from build123d import *

# Parameters (mm, degrees)
PAD_DEPTH    = 6
SKETCH002_R  = 4.2
POCKET_DEPTH = 59.001
CHAMFER_SIZE = 5
FILLET_R     = 16


with BuildPart() as part:
    # Sketch → Pad (new body, symmetric)
    with BuildSketch(Plane.XY):
        with BuildLine():
            Line((20.75, -22.5), (20.75, 22.5))
            Line((20.75, 22.5), (-20.75, 22.5))
            ThreePointArc((-20.75, 22.5), (-33.124369, 17.374369), (-38.25, 5))
            Line((-38.25, 5), (-38.25, -5))
            ThreePointArc((-38.25, -5), (-33.124369, -17.374369), (-20.75, -22.5))
            Line((20.75, -22.5), (-20.75, -22.5))
        make_face()
    extrude(amount=PAD_DEPTH, both=True)

    # Sketch002 → Pocket (cut, through all)
    with BuildSketch(Plane.YZ.offset(20.75)):
        Circle(SKETCH002_R)
    extrude(amount=-POCKET_DEPTH, mode=Mode.SUBTRACT)

    # Chamfer
    chamfer_edges = [part.edges().sort_by_distance(p)[0] for p in [
        (20.75, 22.5, 0),
        (20.75, -22.5, 0),
    ]]
    chamfer(chamfer_edges, length=CHAMFER_SIZE)

    # Fillet
    fillet_edges = [part.edges().sort_by_distance(p)[0] for p in [
        (15.75, 22.5, 0),
        (15.75, -22.5, 0),
    ]]
    fillet(fillet_edges, radius=FILLET_R)


solid = part.part
Read the model definition and answer for the solid it produces. Units are mm, in the model's axes. Coordinates: 2 decimals unless noted, no trailing zeros. Write each loop counter-clockwise with the first axis right and the second up, starting at its lowest first coordinate (ties: lowest second). Pieces come first, ordered by that corner, then holes. Notation, with made-up numbers: (24.5, 53.5) - (80.5, 53.5) arc R8 ccw to (80.5, 58.5) - close; hole circle Ø9 at (35, -36.75). An arc over 180 degrees is marked (long way). One line per question, with ' | ' between items.
Q1. Find section A-A, the plane y = 0. Write down the section's boundary in (x, z), plus the area to 3 significant figures.
Result set:
outline: (-38.25, -6) - (20.75, -6) - (20.75, -4.2) - (-38.25, -4.2) - close; (-38.25, 4.2) - (20.75, 4.2) - (20.75, 6) - (-38.25, 6) - close | area: 212 mm^2
Q2. Find section B-B, the plane z = 0. Write down the section's boundary in (x, y), plus the area to 3 significant figures.
Result set:
outline: (-38.25, -5) arc R17.5 ccw to (-20.75, -22.5) - (9.12, -22.5) arc R16 ccw to (20.44, -17.81) - (20.75, -17.5) - (20.75, -4.2) - (-38.25, -4.2) - close; (-38.25, 4.2) - (20.75, 4.2) - (20.75, 17.5) - (20.44, 17.81) arc R16 ccw to (9.12, 22.5) - (-20.75, 22.5) arc R17.5 ccw to (-38.25, 5) - close | area: 1,990 mm^2
Q3. Consider L1, parallel to Z at x = -12.5, y = 0; L2, parallel to Y at x = 17, z = 2; L3, parallel to Y at x = -32, z = -1.75. Determine where each line is inside the solid, lowest interval first. Write a range as [from, to].
Result set:
L1: [-6, -4.2], [4.2, 6] | L2: [-20.43, -3.69], [3.69, 20.43] | L3: [-18.4, -3.82], [3.82, 18.4]
Q4. Determine the mould class of faces 1 (the cylindrical face through (15.327, -21.248, -0.084)), 2 (the flat face through (-6, 22.5, 0)), 3 (the cylindrical face through (-8.337, 4.006, 1.262)), 4 (the flat face through (20.75, -4.13, 1.42)) for opening direction Y: +Y half, -Y half, draft (parallel to the pull), parting line (faces both ways), or undercut.
Result set:
face 1: -Y half | face 2: +Y half | face 3: undercut | face 4: draft
Q5. Find section C-C, the plane x = -17. Write down the section's boundary in (y, z).
Result set:
outline: (-22.5, -6) - (22.5, -6) - (22.5, 6) - (-22.5, 6) - close; hole circle Ø8.4 at (0, 0)
Q6. Find section D-D, the plane z = -2.75. Write down the section's boundary in (x, y), plus the area to 3 significant figures.
Result set:
outline: (-38.25, -5) arc R17.5 ccw to (-20.75, -22.5) - (9.12, -22.5) arc R16 ccw to (20.44, -17.81) - (20.75, -17.5) - (20.75, -3.17) - (-38.25, -3.17) - close; (-38.25, 3.17) - (20.75, 3.17) - (20.75, 17.5) - (20.44, 17.81) arc R16 ccw to (9.12, 22.5) - (-20.75, 22.5) arc R17.5 ccw to (-38.25, 5) - close | area: 2,110 mm^2
Q7. Each of these flat-tipped pins is pushed along its axis until it touches: P1, Ø6, axis at y = -15.5, z = 2.5, coming from the -X side; P2, Ø4, axis at x = 12, z = -4, coming from the -Y side. Where does it stop, or does it pass through?
Result set:
P1: x = -36.56 | P2: y = -22.48
